Geometry check sheet. Reference: the model listing, model coordinates, mm. Face numbers are marked on the shaded views. A direction names the side the tool comes from. Give positions to 0.01 mm unless a question says otherwise; leave off trailing zeros. Loops run counter-clockwise (first coordinate to the right, second up) from the corner with the lowest first, then second, coordinate; pieces in that order, holes last. Notation, with made-up numbers: (30, 59) - (60, 59) arc R29 ccw to (60, 79) - close; hole circle Ø4 at (7.25, 48.5). An arc over 180 degrees is marked (long way). Use a Markdown table: item, result. Add a question column.
1. Cross-section at A-A on y = 0. Enter the section's corners in (x, z) (3 decimals).
2. Cross-section at B-B on x = 12.7. Enter the section's corners in (y, z) (3 decimals), and give its area (3 significant figures).
3. Depth check by flat-ended pin: P1, Ø1.9, axis at x = -13.5, y = 0.5, coming from the -Z side. Enter the tip coordinate at first touch or a pass-through.
4. Draft check along Y on the marked faces 1, 2 and 3. Enter one of: pulls with the +Y half, pulls with the -Y half, needs draft (parallel to the pull), parting line crosses it, or undercut.
5. Set-up check for the marked faces 4 and 5: record each of +Z, -Z, +X, -X, +Y, -Y from which the full face is reachable in a straight line by a thin tool's end or side.
6. Cross-section at C-C on z = -19. Enter the section's corners in (x, y) (3 decimals), and give its area (3 significant figures).
7. Material ranges on L1, parallel to Y at x = 12.7, z = -22.25 (3 decimals); L2, parallel to X at y = -1, z = -21.75; L3, parallel to Z at x = 0, y = 7.25, recorded low to high.
8. Cross-section at D-D on z = -8.5. Enter the section's corners in (x, y), and give its area (3 significant figures).
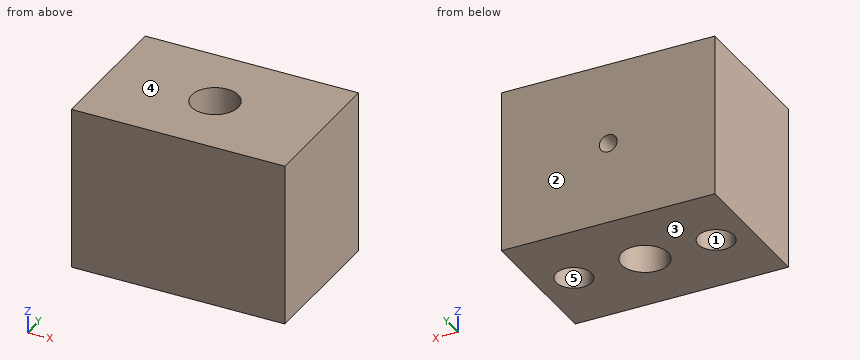
from build123d import *

# Parameters (mm, degrees)
F0_W     = 38.1
F0_H     = 25.4
F0_R     = 4.1656
F1_DEPTH = 29.21
F2_R     = 3.175
F3_DEPTH = 12.7
F4_R     = 1.5875
F5_DEPTH = 12.7


with BuildPart() as f1:
    # F0 (on Top) → F1 (new body)
    with BuildSketch(Plane.XY):
        Rectangle(F0_W, F0_H)
        Circle(F0_R, mode=Mode.SUBTRACT)
    extrude(amount=-F1_DEPTH)

    # F2 (on face) → F3 (cut)
    with BuildSketch(Plane(origin=(0, 0, -29.21), x_dir=(1, 0, 0), z_dir=(0, 0, -1))):
        with Locations((-12.7, 0)):
            Circle(F2_R)
        with Locations((12.7, 0)):
            Circle(F2_R)
    extrude(amount=-F3_DEPTH, mode=Mode.SUBTRACT)

    # F4 (on face) → F5 (cut)
    with BuildSketch(Plane(origin=(0, 12.7, 0), x_dir=(-1, 0, 0), z_dir=(0, 1, 0))):
        with Locations((0, -14.605)):
            Circle(F4_R)
    extrude(amount=-F5_DEPTH, mode=Mode.SUBTRACT)


solid = f1.part
Values found:
| question | item | result |
|---|---|---|
| 1 | outline | (-19.05, -29.21) - (-15.875, -29.21) - (-15.875, -16.51) - (-9.525, -16.51) - (-9.525, -29.21) - (-4.166, -29.21) - (-4.166, 0) - (-19.05, 0) - close; (4.166, -29.21) - (9.525, -29.21) - (9.525, -16.51) - (15.875, -16.51) - (15.875, -29.21) - (19.05, -29.21) - (19.05, 0) - (4.166, 0) - close |
| 2 | outline | (-12.7, -29.21) - (-3.175, -29.21) - (-3.175, -16.51) - (3.175, -16.51) - (3.175, -29.21) - (12.7, -29.21) - (12.7, 0) - (-12.7, 0) - close |
| 2 | area | 661 mm2 |
| 3 | P1 | stops at z = -16.51 |
| 4 | face 1 | undercut |
| 4 | face 2 | pulls with the +Y half |
| 4 | face 3 | needs draft |
| 5 | face 4 | +Z, +X, -X, +Y, -Y |
| 5 | face 5 | -Z |
| 6 | outline | (-19.05, -12.7) - (19.05, -12.7) - (19.05, 12.7) - (-19.05, 12.7) - close; hole circle Ø6.35 at (-12.7, 0); hole circle Ø8.331 at (0, 0); hole circle Ø6.35 at (12.7, 0) |
| 6 | area | 850 mm2 |
| 7 | L1 | y = -12.7 to -3.175, 3.175 to 12.7 |
| 7 | L2 | x = -19.05 to -15.71, -9.69 to -4.04, 4.04 to 9.69, 15.71 to 19.05 |
| 7 | L3 | z = -29.21 to -16.19, -13.02 to 0 |
| 8 | outline | (-19.05, -12.7) - (19.05, -12.7) - (19.05, 12.7) - (-19.05, 12.7) - close; hole circle Ø8.33 at (0, 0) |
| 8 | area | 913 mm2 |
